Could you check a few things on this model? Use its own coordinates, in mm. Face numbers are marked on the shaded views. A direction names the side the tool comes from. Give positions to 0.01 mm unless a question says otherwise; leave off trailing zeros. Loops run counter-clockwise (first coordinate to the right, second up) from the corner with the lowest first, then second, coordinate; pieces in that order, holes last. Notation, with made-up numbers: (57, 28) - (99, 28) arc R20 cw to (99, 58) - close; hole circle Ø2 at (68.5, 77.25). An arc over 180 degrees is marked (long way). Use CSV: the item, a comma, the result in double quotes.
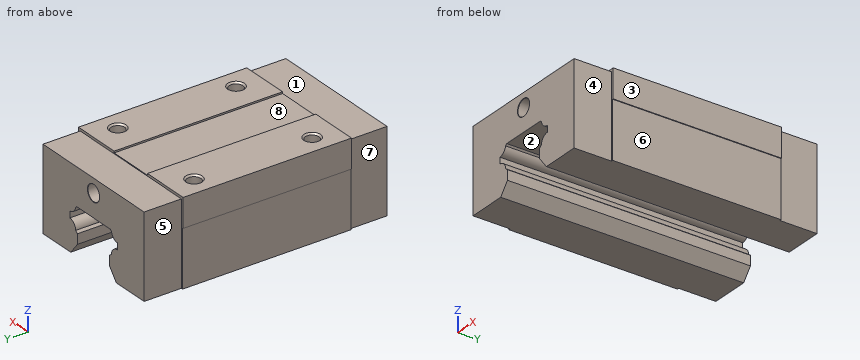
from build123d import *

# Parameters (mm, degrees)
SKIZZE1_W                       = 44
SKIZZE1_H                       = 51.3
AUFSATZ_LINEAR_AUSTRAGEN1_DEPTH = 26
SKIZZE2_W                       = 0.25
SKIZZE2_H                       = 17.25
SCHNITT_LINEAR_AUSTRAGEN1_DEPTH = 64.369472146
SKIZZE3_W                       = 14
SKIZZE3_H                       = 0.5
SCHNITT_LINEAR_AUSTRAGEN2_DEPTH = 64.369472146
SKIZZE4_W                       = 0.25
SKIZZE4_H                       = 17.25
SCHNITT_LINEAR_AUSTRAGEN3_DEPTH = 51.3
SKIZZE5_W                       = 42.5
SKIZZE5_H                       = 25.25
AUFSATZ_LINEAR_AUSTRAGEN2_DEPTH = 11.35
SKIZZE6_W                       = 42.5
SKIZZE6_H                       = 25.25
AUFSATZ_LINEAR_AUSTRAGEN3_DEPTH = 11.35
SCHNITT_LINEAR_AUSTRAGEN4_DEPTH = 83.825116963
BOHRUNG1_D                      = 4.917
BOHRUNG1_DEPTH                  = 15
BOHRUNG1_TIP                    = 1.477215832
BOHRUNG2_D                      = 4.917
BOHRUNG2_DEPTH                  = 15
BOHRUNG2_TIP                    = 1.477215832
DURCHGANGSLOCH_F_R_M3_51_D      = 4.134
DURCHGANGSLOCH_F_R_M3_51_DEPTH  = 6
DURCHGANGSLOCH_F_R_M3_51_TIP    = 1.2419789
FASE1_SIZE                      = 0.483
FASE2_SIZE                      = 0.448979592
FASE3_SIZE                      = 0.0915
FASE4_SIZE                      = 0.448979592


with BuildPart() as part:
    # Skizze1 → Aufsatz-Linear austragen1 (new body)
    with BuildSketch(Plane(origin=(0, 0, 4), x_dir=(-1, 0, 0), z_dir=(0, 0, -1))):
        Rectangle(SKIZZE1_W, SKIZZE1_H)
    extrude(amount=-AUFSATZ_LINEAR_AUSTRAGEN1_DEPTH)

    # Skizze2 → Schnitt-Linear austragen1 (cut, through all)
    with BuildSketch(Plane.XZ.offset(25.65)):
        with Locations((-21.875, 12.625)):
            Rectangle(SKIZZE2_W, SKIZZE2_H)
    extrude(amount=-SCHNITT_LINEAR_AUSTRAGEN1_DEPTH, mode=Mode.SUBTRACT)

    # Skizze3 → Schnitt-Linear austragen2 (cut, through all)
    with BuildSketch(Plane.XZ.offset(25.65)):
        with Locations((0, 29.75)):
            Rectangle(SKIZZE3_W, SKIZZE3_H)
    extrude(amount=-SCHNITT_LINEAR_AUSTRAGEN2_DEPTH, mode=Mode.SUBTRACT)

    # Skizze4 → Schnitt-Linear austragen3 (cut)
    with BuildSketch(Plane.XZ.offset(25.65)):
        with Locations((21.875, 12.625)):
            Rectangle(SKIZZE4_W, SKIZZE4_H)
    extrude(amount=-SCHNITT_LINEAR_AUSTRAGEN3_DEPTH, mode=Mode.SUBTRACT)

    # Skizze5 → Aufsatz-Linear austragen2 (add)
    with BuildSketch(Plane(origin=(0, 25.65, 0), x_dir=(-1, 0, 0), z_dir=(0, 1, 0))):
        with Locations((0, 16.625)):
            Rectangle(SKIZZE5_W, SKIZZE5_H)
    extrude(amount=AUFSATZ_LINEAR_AUSTRAGEN2_DEPTH)

    # Skizze6 → Aufsatz-Linear austragen3 (add)
    with BuildSketch(Plane.XZ.offset(25.65)):
        with Locations((0, 16.625)):
            Rectangle(SKIZZE6_W, SKIZZE6_H)
    extrude(amount=AUFSATZ_LINEAR_AUSTRAGEN3_DEPTH)

    # Skizze7 → Schnitt-Linear austragen4 (cut, through all)
    with BuildSketch(Plane.XZ.offset(37)):
        with BuildLine():
            Line((-9.59375, 4), (9.59375, 4))
            Line((9.59375, 4), (6.75, 7.5))
            Line((6.75, 7.5), (6.75, 10.5))
            Line((6.75, 10.5), (7.5, 11.109375))
            ThreePointArc((7.5, 11.109375), (8.270470592, 12.806156162), (10, 13.5))
            Line((10, 13.5), (10, 15.5))
            ThreePointArc((10, 15.5), (8.232233047, 16.232233047), (7.5, 18))
            Line((7.5, 18), (-7.5, 18))
            ThreePointArc((-7.5, 18), (-8.232233047, 16.232233047), (-10, 15.5))
            Line((-10, 15.5), (-10, 13.5))
            ThreePointArc((-10, 13.5), (-8.270470592, 12.806156162), (-7.5, 11.109375))
            Line((-7.5, 11.109375), (-6.75, 10.5))
            Line((-6.75, 10.5), (-6.75, 7.5))
            Line((-6.75, 7.5), (-9.59375, 4))
        make_face()
    extrude(amount=-SCHNITT_LINEAR_AUSTRAGEN4_DEPTH, mode=Mode.SUBTRACT)

    # Bohrung1
    with Locations(Plane(origin=(0, -37, 0), x_dir=(-1, 0, 0), z_dir=(0, -1, 0))):
        with Locations((0, -25)):
            Hole(BOHRUNG1_D / 2, depth=BOHRUNG1_DEPTH)
            with Locations((0, 0, -(BOHRUNG1_DEPTH + BOHRUNG1_TIP / 2))):  # 118° drill point
                Cone(0, BOHRUNG1_D / 2, BOHRUNG1_TIP, mode=Mode.SUBTRACT)

    # Bohrung2
    with Locations(Plane(origin=(0, 37, 0), x_dir=(1, 0, 0), z_dir=(0, 1, 0))):
        with Locations((0, -25)):
            Hole(BOHRUNG2_D / 2, depth=BOHRUNG2_DEPTH)
            with Locations((0, 0, -(BOHRUNG2_DEPTH + BOHRUNG2_TIP / 2))):  # 118° drill point
                Cone(0, BOHRUNG2_D / 2, BOHRUNG2_TIP, mode=Mode.SUBTRACT)

    # Durchgangsloch für M3.51
    with Locations(Plane.XY.offset(30)):
        with Locations((16, -18), (16, 18), (-16, 18), (-16, -18)):
            Hole(DURCHGANGSLOCH_F_R_M3_51_D / 2, depth=DURCHGANGSLOCH_F_R_M3_51_DEPTH)
            with Locations((0, 0, -(DURCHGANGSLOCH_F_R_M3_51_DEPTH + DURCHGANGSLOCH_F_R_M3_51_TIP / 2))):  # 118° drill point
                Cone(0, DURCHGANGSLOCH_F_R_M3_51_D / 2, DURCHGANGSLOCH_F_R_M3_51_TIP, mode=Mode.SUBTRACT)

    # Fase1
    fase1_edges = [part.edges().sort_by_distance(p)[0] for p in [
        (-13.933, -18, 30),
        (-13.933, 18, 30),
        (18.067, 18, 30),
        (18.067, -18, 30),
    ]]
    chamfer(fase1_edges, length=FASE1_SIZE)

    # Fase2
    # the kernel refuses this chamfer: 0.448979592, 0.406117321 mm, written as the material it adds along each edge
    with BuildSketch(Plane(origin=(-7.5, -37, 18), x_dir=(1, 0, 0), z_dir=(0, 1, 0))) as fase2_piece_1:
        with BuildLine():
            Line((FASE2_SIZE, 0), (-0.03932739, 0.441690284))
            ThreePointArc((-0.03932739, 0.441690284), (-0.010448273, 0.22832477), (0, 0))
            Line((0, 0), (FASE2_SIZE, 0))
        make_face()
    extrude(amount=74)

    # Fase3
    fase3_edges = [part.edges().sort_by_distance(p)[0] for p in [
        (-2.4585, -37, 25),
        (2.4585, 37, 25),
    ]]
    chamfer(fase3_edges, length=FASE3_SIZE)

    # Fase4
    # the kernel refuses this chamfer: 0.448979592, 0.406117321 mm, written as the material it adds along each edge
    with BuildSketch(Plane(origin=(7.5, -37, 18), x_dir=(0.08868753028202897, 0, -0.9960594972050988), z_dir=(0, 1, 0))) as fase4_piece_1:
        with BuildLine():
            Line((0.443437651, 0), (-FASE4_SIZE * 0.0886875302498, FASE4_SIZE * 0.996059496843))
            Line((-FASE4_SIZE * 0.0886875302498, FASE4_SIZE * 0.996059496843), (0, 0))
            ThreePointArc((0, 0), (0.228351687, 0.009842458), (0.443437651, 0))
        make_face()
    extrude(amount=74)


solid = part.part
1) Which directions (+Z, -Z, +X, -X, +Y, -Y) give clear straight access to the entire face, cutting with the end or side of a thin tool? Please do the marked faces 4, 5, 6, 7 and 8.
Answer below:
face 4,"+Z, -Z, +X, -Y"
face 5,"+Z, -Z, -X, +Y"
face 6,"-Z, +X, +Y, -Y"
face 7,"+Z, -Z, -X, -Y"
face 8,"+Z, +Y, -Y"
2) Suppose I cut it at D-D (x = 5). Please give me the cut outline in (y, z), plus the area to 3 significant figures.
Answer below:
outline,"(-37, 18) - (37, 18) - (37, 29.25) - (25.65, 29.25) - (25.65, 29.5) - (-25.65, 29.5) - (-25.65, 29.25) - (-37, 29.25) - close"
area,"845 mm2"
3) We'd pull the mould along X, two halves only. Please class the marked faces 1, 2 and 3: +X half, -X half, draft (parallel to the pull), parting line (faces both ways), or undercut.
Answer below:
face 1,"draft"
face 2,"undercut"
face 3,"+X half"
4) Suppose I cut it at A-A (z = 8.5). Please give me the cut outline in (x, y).
Answer below:
outline,"(-21.75, -25.65) - (-21.25, -25.65) - (-21.25, -37) - (-6.75, -37) - (-6.75, 37) - (-21.25, 37) - (-21.25, 25.65) - (-21.75, 25.65) - close; (6.75, -37) - (21.25, -37) - (21.25, -25.65) - (21.75, -25.65) - (21.75, 25.65) - (21.25, 25.65) - (21.25, 37) - (6.75, 37) - close"
5) I'm going to push flat-ended pins straight in: P1, Ø12, axis at x = -3, y = -10.5, coming from the -Z side; P2, Ø5, axis at x = 16, y = 18, coming from the +Z side; P3, Ø7, axis at x = 0.5, y = -3, coming from the -Z side. Where does each tip first touch, or does it pass through?
Answer below:
P1,"stops at z = 4.73"
P2,"stops at z = 29.95"
P3,"stops at z = 18"
6) I need wall thicknesses on line 1 along X through (y, z) = (18, 26.6); line 2 along Y through (x, z) = (16, 27.6); line 3 along X through (y, z) = (-22.5, 25.25). Which ranges of each line are inside material? Lowest first, please.
Answer below:
line 1,"x = -22 to -18.07, -13.93 to 13.93, 18.07 to 22"
line 2,"y = -37 to -20.07, -15.93 to 15.93, 20.07 to 37"
line 3,"x = -22 to -2.45, 2.45 to 22"
